Build history of the part. All positions in model axes, mm. Face numbers are marked on the shaded views. A direction names the side the tool comes from. Give positions to 0.01 mm unless a question says otherwise; leave off trailing zeros. Write each loop counter-clockwise with the first axis right and the second up, starting at its lowest first coordinate (ties: lowest second). Pieces come first, ordered by that corner, then holes. Notation, with made-up numbers: (14, 85.5) -> (25, 85.5) arc R37 cw to (25, 121.5) -> close; hole circle Ø5 at (30.25, -13). An arc over 180 degrees is marked (long way). Put each result on its own line as item: value.
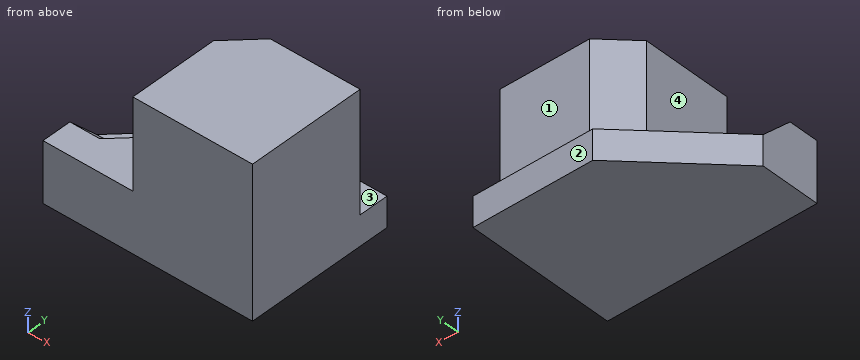
from build123d import *

# Parameters (mm, degrees)
SKETCH1_W           = 70
SKETCH1_H           = 50
BOSS_EXTRUDE1_DEPTH = 50
CUT_EXTRUDE1_DEPTH  = 50
SKETCH3_W           = 40
SKETCH3_H           = 10
CUT_EXTRUDE2_DEPTH  = 50
CUT_EXTRUDE3_DEPTH  = 20
CUT_EXTRUDE4_DEPTH  = 10
CUT_EXTRUDE6_DEPTH  = 30
CUT_EXTRUDE7_DEPTH  = 30
CUT_EXTRUDE9_DEPTH  = 10
BOSS_EXTRUDE2_DEPTH = 43
CUT_EXTRUDE10_DEPTH = 10


with BuildPart() as part:
    # Sketch1 → Boss-Extrude1 (new body)
    with BuildSketch(Plane.XY):
        with Locations((35, 25)):
            Rectangle(SKETCH1_W, SKETCH1_H)
    extrude(amount=BOSS_EXTRUDE1_DEPTH)

    # Sketch2 → Cut-Extrude1 (cut)
    with BuildSketch(Plane.XY.offset(50)):
        Polygon((0, 20), (30, 50), (0, 50), align=None)
    extrude(amount=-CUT_EXTRUDE1_DEPTH, mode=Mode.SUBTRACT)

    # Sketch3 → Cut-Extrude2 (cut)
    with BuildSketch(Plane(origin=(70, 0, 0), x_dir=(0, 0, -1), z_dir=(1, 0, 0))):
        with Locations((-30, 45)):
            Rectangle(SKETCH3_W, SKETCH3_H)
    extrude(amount=-CUT_EXTRUDE2_DEPTH, mode=Mode.SUBTRACT)

    # Sketch4 → Cut-Extrude3 (cut)
    with BuildSketch(Plane.XY.offset(50)):
        Polygon((30, 30), (40, 40), (20, 40), (0, 20), (0, 0), (30, 0), align=None)
    extrude(amount=-CUT_EXTRUDE3_DEPTH, mode=Mode.SUBTRACT)

    # Sketch5 → Cut-Extrude4 (cut)
    with BuildSketch(Plane.XY.offset(30)):
        Polygon((0, 10), (10, 10), (40, 40), (20, 40), (0, 20), align=None)
    extrude(amount=-CUT_EXTRUDE4_DEPTH, mode=Mode.SUBTRACT)

    # Sketch6 → Cut-Extrude6 (cut)
    with BuildSketch(Plane.ZY):
        Polygon((30, 10), (20, 0), (30, 0), align=None)
    extrude(amount=-CUT_EXTRUDE6_DEPTH, mode=Mode.SUBTRACT)

    # Sketch7 → Cut-Extrude7 (cut)
    with BuildSketch(Plane.ZY):
        Polygon((30, 10), (20, 10), (20, 0), align=None)
    extrude(amount=-CUT_EXTRUDE7_DEPTH, mode=Mode.SUBTRACT)

    # Sketch9 → Cut-Extrude9 (cut)
    with BuildSketch(Plane.XY.offset(20)):
        Polygon((20, 40), (40, 40), (10, 10), (0, 10), (0, 20), align=None)
    extrude(amount=-CUT_EXTRUDE9_DEPTH, mode=Mode.SUBTRACT)

    # Sketch10 → Boss-Extrude2 (add)
    with BuildSketch(Plane.ZY):
        Polygon((10, 20), (20, 10), (10, 10), align=None)
    extrude(amount=-BOSS_EXTRUDE2_DEPTH)

    # Sketch13 → Cut-Extrude10 (cut)
    with BuildSketch(Plane.XY.offset(30)):
        Polygon((10, 10), (30, 10), (30, 30), align=None)
    extrude(amount=-CUT_EXTRUDE10_DEPTH, mode=Mode.SUBTRACT)


solid = part.part
1) Slice it at A-A (y = 29). Write the cut outline in (x, z).
Filled sheet:
outline: (9, 0) -> (70, 0) -> (70, 50) -> (30, 50) -> (30, 20) -> (29, 20) -> (29, 10) -> (9, 10) -> close
2) Slice it at B-B (x = 16). Write the cut outline in (y, z), plus the area to 3 significant figures.
Filled sheet:
outline: (0, 0) -> (36, 0) -> (36, 10) -> (20, 10) -> (16, 14) -> (16, 20) -> (0, 20) -> close
area: 528 mm2
3) Wall check: L1, parallel to X at y = 3, z = 38.5; L2, parallel to Z at x = 22.5, y = 4.5; L3, parallel to Z at x = 12, y = 26.5. Give the ranges that are in metal, low to high.
Filled sheet:
L1: 30 to 70
L2: 0 to 20
L3: 0 to 10
4) Slice it at D-D (y = 22). Write the cut outline in (x, z), plus the area to 3 significant figures.
Filled sheet:
outline: (2, 0) -> (70, 0) -> (70, 50) -> (30, 50) -> (30, 20) -> (22, 20) -> (22, 10) -> (2, 10) -> close
area: 2,360 mm2
5) Slice it at C-C (z = 39). Write the cut outline in (x, y), plus the area to 3 significant figures.
Filled sheet:
outline: (30, 0) -> (70, 0) -> (70, 40) -> (40, 40) -> (30, 30) -> close
area: 1,550 mm2
6) Tool access for the marked faces 1, 2, 3 and 4: list every direction of +Z, -Z, +X, -X, +Y, -Y with a clear straight run to the whole face (end or side of a thin tool).
Filled sheet:
face 1: +Z, +X, -X, +Y
face 2: +Z, -Z, +X, -X, +Y
face 3: +Z, -X, +Y
face 4: +Z, -X, +Y, -Y
7) Pin check, flat tips, straight feed: pin 1 (10 mm diameter, centred on x = 51.5, z = 28.5, fed in from +Y); pin 2 (10 mm diameter, centred on x = 8, y = 32.5, fed in from +Z). Stop position of each tip, or through.
Filled sheet:
pin 1: y = 40
pin 2: z = 10
